Verification items for the finished model (mm, model axes). A direction names the side the tool comes from. Round coordinates to 2 decimals unless told otherwise and drop trailing zeros. Write each loop counter-clockwise with the first axis right and the second up, starting at its lowest first coordinate (ties: lowest second). Pieces come first, ordered by that corner, then holes.
from build123d import *

# Parameters (mm, degrees)
F1_DEPTH = 30
F3_DEPTH = 20.001
F4_W     = 20
F4_H     = 10
F5_DEPTH = 10


with BuildPart() as f1:
    # F0 (on Right) → F1 (new body, symmetric)
    with BuildSketch(Plane.YZ):
        Polygon((-30, 0), (0, 0), (0, 40), (-20, 40), (-20, 10), (-30, 10), align=None)
    extrude(amount=F1_DEPTH, both=True)

    # F2 (on face) → F3 (cut, through all)
    with BuildSketch(Plane.XZ.offset(20)):
        with BuildLine():
            Line((20, 40), (-20, 40))
            ThreePointArc((-20, 40), (0, 20), (20, 40))
        make_face()
    extrude(amount=-F3_DEPTH, mode=Mode.SUBTRACT)

    # F4 (on face) → F5 (join)
    with BuildSketch(Plane.XZ.offset(30)):
        with Locations((0, 5)):
            Rectangle(F4_W, F4_H)
        with Locations((0, 15)):
            Rectangle(F4_W, F4_H)
    extrude(amount=F5_DEPTH)


solid = f1.part
Q1. Sectioned sample at A-A (z = 13). Enter the section's corners in (x, y).
Recorded:
outline: (-30, -20) - (30, -20) - (30, 0) - (-30, 0) - close; (-10, -40) - (10, -40) - (10, -30) - (-10, -30) - close
Q2. Tool access check on faces 5 (the flat face through (0, -15, 0)), 6 (the flat face through (10, -35, 10)), 7 (the flat face through (0, -25, 10)), 8 (the flat face through (-10, -35, 10)). Record the directions out of +Z, -Z, +X, -X, +Y, -Y that give a thin tool (end or side, any length) a straight path to the whole face; none if there is none.
Recorded:
face 5: -Z, +X, -X, +Y, -Y
face 6: +Z, -Z, +X, -Y
face 7: +Z, +X, -X
face 8: +Z, -Z, -X, -Y
Q3. Depth check by flat-ended pin: P1, Ø8, axis at x = -4, y = -26.5, coming from the +Z side; P2, Ø1, axis at x = -10.5, z = 5.5, coming from the +Y side; P3, Ø5, axis at y = -32.5, z = 12, coming from the +X side; P4, Ø3, axis at x = 16.5, z = 3, coming from the -Y side. Enter the tip coordinate at first touch or a pass-through.
Recorded:
P1: stops at z = 20
P2: stops at y = 0
P3: stops at x = 10
P4: stops at y = -30
Q4. Sectioned sample at D-D (x = -24). Enter the section's corners in (y, z).
Recorded:
outline: (-30, 0) - (0, 0) - (0, 40) - (-20, 40) - (-20, 10) - (-30, 10) - close
Q5. Sectioned sample at C-C (y = -4). Enter the section's corners in (x, z), plus the area to 3 significant figures.
Recorded:
outline: (-30, 0) - (30, 0) - (30, 40) - (20, 40) arc R20 cw to (-20, 40) - (-30, 40) - close
area: 1,770 mm2
Q6. Material ranges on line 1 along Y through (x, z) = (19.5, 13); line 2 along Z through (x, y) = (-6, -36.5); line 3 along Z through (x, y) = (9, -23), recorded low to high.
Recorded:
line 1: y = -20 to 0
line 2: z = 0 to 20
line 3: z = 0 to 10
Q7. Release check for a two-part mould opening along Y. For faces 1 (the flat face through (0, -20, 19)), 2 (the flat face through (0, -35, 20)), 3 (the flat face through (0, 0, 15)), 4 (the flat face through (0, -30, 15)) record: released by +Y, released by -Y, zero draft, split by the parting line, or undercut.
Recorded:
face 1: undercut
face 2: zero draft
face 3: released by +Y
face 4: undercut
Q8. Sectioned sample at B-B (x = 0). Enter the section's corners in (y, z).
Recorded:
outline: (-40, 0) - (0, 0) - (0, 20) - (-20, 20) - (-20, 10) - (-30, 10) - (-30, 20) - (-40, 20) - close
